Part model, mm, in its own coordinate system. A direction names the side the tool comes from. Coordinates: 2 decimals unless noted, no trailing zeros. Write each loop counter-clockwise with the first axis right and the second up, starting at its lowest first coordinate (ties: lowest second). Pieces come first, ordered by that corner, then holes. Notation, with made-up numbers: (25, 63.25) - (66, 63.25) arc R31 cw to (66, 100.25) - close; hole circle Ø8 at (41, -35.75). An arc over 180 degrees is marked (long way). Use a Markdown table: item, result.
```python
from build123d import *

# Parameters (mm, degrees)
SKETCH1_W           = 100
SKETCH1_H           = 80
BOSS_EXTRUDE2_DEPTH = 2
SKETCH3_W           = 96
SKETCH3_H           = 76
BOSS_EXTRUDE3_DEPTH = 1.5
SKETCH5_R           = 2
CUT_EXTRUDE1_DEPTH  = 35
SHELL1_START        = 2
SHELL1_DEPTH        = 1.5
FILLET1_R           = 4
FILLET2_R           = 4
FILLET3_R           = 4
SKETCH10_R          = 2
SKETCH10_W          = 5.536600299
SKETCH10_H          = 4
SKETCH10_H_2        = 4.208329991
SKETCH10_H_3        = 3.982444476
CUT_EXTRUDE2_DEPTH  = 5
SKETCH11_R          = 2.6
CUT_EXTRUDE3_DEPTH  = 2


# Read off the part's stored shape, not the designer's step: Shell1
with BuildPart() as part:
    # Sketch1 → Boss-Extrude2 (new body)
    with BuildSketch(Plane(origin=(0, 0, 0), x_dir=(1, 0, 0), z_dir=(0, 1, 0))):
        Rectangle(SKETCH1_W, SKETCH1_H)
    extrude(amount=BOSS_EXTRUDE2_DEPTH)

    # Sketch3 → Boss-Extrude3 (add)
    with BuildSketch(Plane(origin=(0, 2, 0), x_dir=(1, 0, 0), z_dir=(0, 1, 0))):
        Rectangle(SKETCH3_W, SKETCH3_H)
    extrude(amount=BOSS_EXTRUDE3_DEPTH)

    # Sketch5 → Cut-Extrude1 (cut)
    with BuildSketch(Plane(origin=(0, 3.5, 0), x_dir=(1, 0, 0), z_dir=(0, 1, 0))):
        with Locations(Location((-43, -33, 0), (0, 0, 270))):
            Circle(SKETCH5_R)
        with Locations(Location((-43, 33, 0), (0, 0, 270))):
            Circle(SKETCH5_R)
        with Locations(Location((43, -33, 0), (0, 0, 270))):
            Circle(SKETCH5_R)
        with Locations(Location((43, 33, 0), (0, 0, 270))):
            Circle(SKETCH5_R)
    extrude(amount=-CUT_EXTRUDE1_DEPTH, mode=Mode.SUBTRACT)

    # Shell1 outline → Shell1 (cut)
    with BuildSketch(Plane(origin=(0, 0, 0), x_dir=(1, 0, 0), z_dir=(0, 1, 0)).offset(SHELL1_START)):
        with BuildLine():
            ThreePointArc((-46, 35.645751311), (-45.828427125, 35.828427125), (-45.645751311, 36))
            Line((-45.645751311, 36), (-46, 36))
            Line((-46, 36), (-46, 35.645751311))
        make_face()
        with BuildLine():
            ThreePointArc((-40.354248689, 36), (-40.171572875, 30.171572875), (-46, 30.354248689))
            Line((-46, 30.354248689), (-46, -30.354248689))
            ThreePointArc((-46, -30.354248689), (-40.171572875, -30.171572875), (-40.354248689, -36))
            Line((-40.354248689, -36), (40.354248689, -36))
            ThreePointArc((40.354248689, -36), (40.171572875, -30.171572875), (46, -30.354248689))
            Line((46, -30.354248689), (46, 30.354248689))
            ThreePointArc((46, 30.354248689), (40.171572875, 30.171572875), (40.354248689, 36))
            Line((40.354248689, 36), (-40.354248689, 36))
        make_face()
        with BuildLine():
            Line((46, 36), (45.645751311, 36))
            ThreePointArc((45.645751311, 36), (45.828427125, 35.828427125), (46, 35.645751311))
            Line((46, 35.645751311), (46, 36))
        make_face()
        with BuildLine():
            Line((-46, -35.645751311), (-46, -36))
            Line((-46, -36), (-45.645751311, -36))
            ThreePointArc((-45.645751311, -36), (-45.828427125, -35.828427125), (-46, -35.645751311))
        make_face()
        with BuildLine():
            ThreePointArc((46, -35.645751311), (45.828427125, -35.828427125), (45.645751311, -36))
            Line((45.645751311, -36), (46, -36))
            Line((46, -36), (46, -35.645751311))
        make_face()
    extrude(amount=SHELL1_DEPTH, mode=Mode.SUBTRACT)

    # Fillet1
    fillet1_edges = [part.edges().sort_by_distance(p)[0] for p in [
        (-48, 2.75, 38),
    ]]
    fillet(fillet1_edges, radius=FILLET1_R)

    # Fillet2
    fillet2_edges = [part.edges().sort_by_distance(p)[0] for p in [
        (48, 2.75, 38),
        (48, 2.75, -38),
        (-48, 2.75, -38),
    ]]
    fillet(fillet2_edges, radius=FILLET2_R)

    # Fillet3
    fillet3_edges = [part.edges().sort_by_distance(p)[0] for p in [
        (-50, 1, -40),
        (50, 1, -40),
        (50, 1, 40),
        (-50, 1, 40),
    ]]
    fillet(fillet3_edges, radius=FILLET3_R)

    # Sketch10 → Cut-Extrude2 (cut)
    with BuildSketch(Plane.XZ):
        with Locations(Location((0, -11, 0), (0, 0, 270))):
            Circle(SKETCH10_R)
        with Locations(Location((0, 0, 0), (0, 0, 270))):
            Circle(SKETCH10_R)
        with Locations(Location((0, 11, 0), (0, 0, 270))):
            Circle(SKETCH10_R)
        with Locations(Location((20, 0, 0), (0, 0, 270))):
            Circle(SKETCH10_R)
        with Locations((-18.761111615, -11.119893759)):
            Rectangle(SKETCH10_W, SKETCH10_H)
        with Locations((-18.761111615, -0.119893758)):
            Rectangle(SKETCH10_W, SKETCH10_H_2)
        with Locations((-18.761111615, 10.880106241)):
            Rectangle(SKETCH10_W, SKETCH10_H_3)
    extrude(amount=-CUT_EXTRUDE2_DEPTH, mode=Mode.SUBTRACT)

    # Sketch11 → Cut-Extrude3 (cut)
    with BuildSketch(Plane.XZ):
        with Locations(Location((43, 33, 0), (0, 0, 270))):
            Circle(SKETCH11_R)
        with Locations(Location((43, -33, 0), (0, 0, 270))):
            Circle(SKETCH11_R)
        with Locations(Location((-43, -33, 0), (0, 0, 270))):
            Circle(SKETCH11_R)
        with Locations(Location((-43, 33, 0), (0, 0, 270))):
            Circle(SKETCH11_R)
    extrude(amount=-CUT_EXTRUDE3_DEPTH, mode=Mode.SUBTRACT)


solid = part.part
```
Item 1: Band-saw the part on C-C, the plane x = -19.5. Give the cut face in (y, z).
From the geometry:
| item | result |
|---|---|
| outline | (0, -40) - (2, -40) - (2, -38) - (3.5, -38) - (3.5, -36) - (2, -36) - (2, -13.12) - (0, -13.12) - close; (0, -9.12) - (2, -9.12) - (2, -2.22) - (0, -2.22) - close; (0, 1.98) - (2, 1.98) - (2, 8.89) - (0, 8.89) - close; (0, 12.87) - (2, 12.87) - (2, 36) - (3.5, 36) - (3.5, 38) - (2, 38) - (2, 40) - (0, 40) - close |
Item 2: Drill centre lines: probe 1 along X at (y, z) = (2.65, 33); probe 2 along X at (y, z) = (0.7, 0); probe 3 along Z at (x, y) = (0, 2.4). Where is each one in solid material? Low to high.
From the geometry:
| item | result |
|---|---|
| probe 1 | -48 to -45, -41 to -39, 39 to 41, 45 to 48 |
| probe 2 | -50 to -21.53, -15.99 to -2, 2 to 18, 22 to 50 |
| probe 3 | -38 to -36, 36 to 38 |
Item 3: Which spindle directions (+Z, -Z, +X, -X, +Y, -Y) get a long thin tool onto all of the face, cutting with end or side? Do faces 1 (the face through (-15.993, 1, -11)), 2 (the face through (-48.859, 1.014, -38.797)), 3 (the face through (46.859, 2.76, -36.797)), 4 (the face through (-46.797, 2.76, 36.859)), 5 (the face through (41, 2, 32)). Say none if no direction does.
From the geometry:
| item | result |
|---|---|
| face 1 | +Y, -Y |
| face 2 | -Z, -X, +Y, -Y |
| face 3 | -Z, +X, +Y |
| face 4 | +Z, -X, +Y |
| face 5 | -Y |
Item 4: Band-saw the part on D-D, the plane z = -11. Give the cut face in (x, y), then the cut area to 3 significant figures.
From the geometry:
| item | result |
|---|---|
| outline | (-50, 0) - (-21.53, 0) - (-21.53, 2) - (-46, 2) - (-46, 3.5) - (-48, 3.5) - (-48, 2) - (-50, 2) - close; (-15.99, 0) - (-2, 0) - (-2, 2) - (-15.99, 2) - close; (2, 0) - (50, 0) - (50, 2) - (48, 2) - (48, 3.5) - (46, 3.5) - (46, 2) - (2, 2) - close |
| area | 187 mm^2 |
Item 5: Band-saw the part on B-B, the plane y = 1.15. Count the separate pieces of the cut face and the enclosed holes in it, then the cut area to 3 significant figures.
From the geometry:
| item | result |
|---|---|
| separate pieces | 1 |
| enclosed holes | 11 |
| area | 7,780 mm^2 |
Item 6: Band-saw the part on A-A, the plane z = 0. Give the cut face in (x, y), then the cut area to 3 significant figures.
From the geometry:
| item | result |
|---|---|
| outline | (-50, 0) - (-21.53, 0) - (-21.53, 2) - (-46, 2) - (-46, 3.5) - (-48, 3.5) - (-48, 2) - (-50, 2) - close; (-15.99, 0) - (-2, 0) - (-2, 2) - (-15.99, 2) - close; (2, 0) - (18, 0) - (18, 2) - (2, 2) - close; (22, 0) - (50, 0) - (50, 2) - (48, 2) - (48, 3.5) - (46, 3.5) - (46, 2) - (22, 2) - close |
| area | 179 mm^2 |
Item 7: Drop flat-ended pins along their axis: P1, Ø4, axis at x = 32, z = 15.5, coming from the +Y side; P2, Ø1.6, axis at x = 43, z = -33.5, coming from the -Y side; P3, Ø0.8, axis at y = 3, z = -15, coming from the -X side. Give the stop position or say it passes through.
From the geometry:
| item | result |
|---|---|
| P1 | y = 2 |
| P2 | through |
| P3 | x = -48 |
